Geometry: see drawing. Coordinates: mm, zero at the bounding-box minimum. A direction names the side the tool comes from. Coordinates: 2 decimals unless noted, no trailing zeros. Write each loop counter-clockwise with the first axis right and the second up, starting at its lowest first coordinate (ties: lowest second). Pieces come first, ordered by that corner, then holes. Notation, with made-up numbers: M 53.25,46.5 L 90.25,46.5 A19 ccw 90.25,61.5 Z; hole C 53,-13 d10. An arc over 180 degrees is marked long. Answer as CSV lines item,"result". Start each with the question number.
1. Section D-D on z = 4. Return the cut outline in (x, y).
2. Reachability of the marked faces 1, 2 and 3 from +Z, -Z, +X, -X, +Y, -Y: full face, straight path, thin tool, end or side. Return the list, or none.
3. Contact query for flat-ended pins moving along their axis: pin 1 Ø5 at (x, y) = (26, 47.5) entering from +Z; pin 2 Ø1.8 at (y, z) = (13, 42) entering from -X; pin 3 Ø10 at (x, z) = (35, 37) entering from +Y; pin 4 Ø3.5 at (x, y) = (40.5, 58) entering from +Z. Output: stop coordinate, or through.
4. Line query: probe 1 along Y at (x, z) = (40.4, 42) (3 decimals); probe 2 along X at (y, z) = (16, 13); probe 3 along Y at (x, z) = (41.15, 42) (3 decimals). Output: solid intervals per line, ascending. Write a range as [from, to].
5. Section B-B on z = 42. Return the cut outline in (x, y) (3 decimals), plus the area to 3 significant figures.
6. Section C-C on y = 60. Return the cut outline in (x, z), plus the area to 3 significant figures.
7. Section A-A on z = 11. Return the cut outline in (x, y).
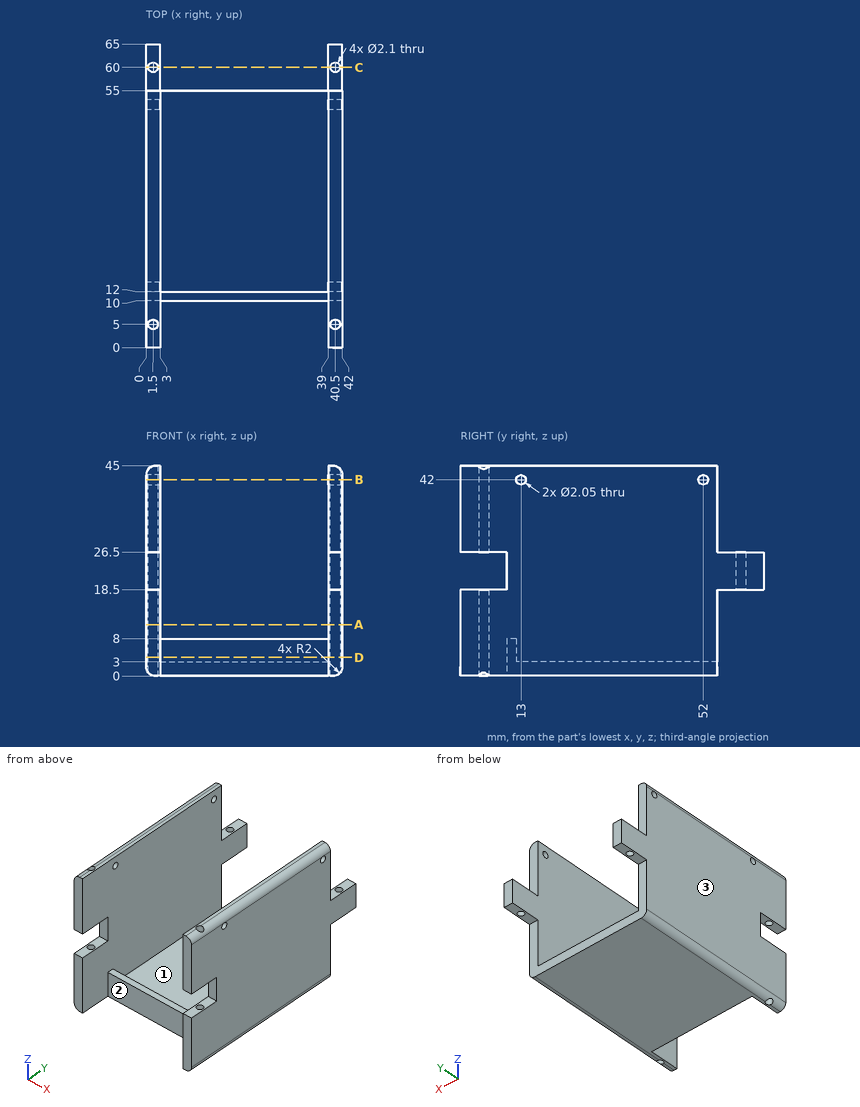
Values:
1,outline,"M 0,0 L 3,0 L 3,10 L 39,10 L 39,0 L 42,0 L 42,55 L 39,55 L 39,12 L 3,12 L 3,55 L 0,55 Z; hole C 1.5,5 d2.1; hole C 40.5,5 d2.1"
2,face 1,"+Z, +Y"
2,face 2,"+Z, -Z, -Y"
2,face 3,"+Z, -Z, -X, +Y, -Y"
3,pin 1,"z = 3"
3,pin 2,"through"
3,pin 3,"y = 55"
3,pin 4,"z = 26.5"
4,probe 1,"[0, 3.955], [6.045, 11.975], [14.025, 50.975], [53.025, 55]"
4,probe 2,"[0, 3], [39, 42]"
4,probe 3,"[0, 4.175], [5.825, 11.975], [14.025, 50.975], [53.025, 55]"
5,outline,"M 0,0 L 3,0 L 3,11.975 L 0,11.975 Z; M 0,14.025 L 3,14.025 L 3,50.975 L 0,50.975 Z; M 0,53.025 L 3,53.025 L 3,55 L 0,55 Z; M 39,0 L 42,0 L 42,11.975 L 39,11.975 Z; M 39,14.025 L 42,14.025 L 42,50.975 L 39,50.975 Z; M 39,53.025 L 42,53.025 L 42,55 L 39,55 Z; hole C 1.5,5 d2.1; hole C 40.5,5 d2.1"
5,area,"298 mm²"
6,outline,"M 0,18.5 L 0.45,18.5 L 0.45,26.5 L 0,26.5 Z; M 2.55,18.5 L 3,18.5 L 3,26.5 L 2.55,26.5 Z; M 39,18.5 L 39.45,18.5 L 39.45,26.5 L 39,26.5 Z; M 41.55,18.5 L 42,18.5 L 42,26.5 L 41.55,26.5 Z"
6,area,"14.4 mm²"
7,outline,"M 0,0 L 3,0 L 3,55 L 0,55 Z; M 39,0 L 42,0 L 42,55 L 39,55 Z; hole C 1.5,5 d2.1; hole C 40.5,5 d2.1"
